Build history of the part. All positions in model axes, mm. Face numbers are marked on the shaded views. A direction names the side the tool comes from. Round coordinates to 2 decimals unless told otherwise and drop trailing zeros. Loops run counter-clockwise (first coordinate to the right, second up) from the corner with the lowest first, then second, coordinate; pieces in that order, holes last. Notation, with made-up numbers: M 21,-9 L 28,-9 A36 cw 28,27 Z; hole C 8.5,-35 d3. An arc over 180 degrees is marked long. One line per item, written item: value.
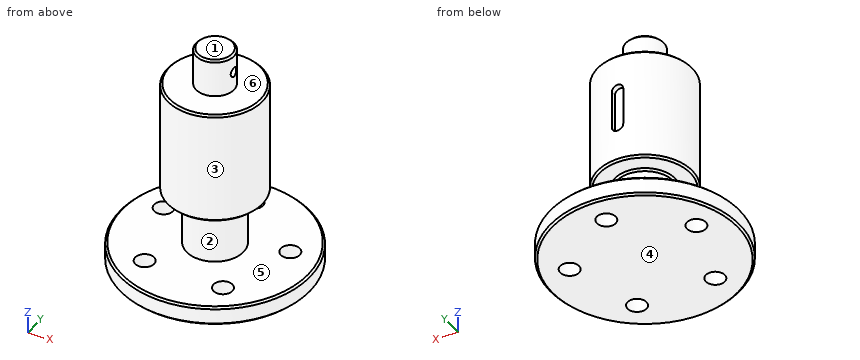
```python
from build123d import *

# Parameters (mm, degrees)
SKETCH_1_R              = 50
EXTRUDE_1_DEPTH         = 10
SKETCH_2_R              = 15
EXTRUDE_2_DEPTH         = 28
SKETCH_3_R              = 16
EXTRUDE_3_DEPTH         = 2
SKETCH_4_R              = 25
EXTRUDE_4_DEPTH         = 60
SKETCH_5_R              = 10
EXTRUDE_5_DEPTH         = 20
CHAMFER_1_SIZE          = 1
HOLE_WIZARD_10_0_10_1_D = 10
CUT_EXTRUDE_1_DEPTH     = 3
HOLE_WIZARD_5_0_5_1_D   = 5


# Read off the part's stored shape, not the designer's step: 구배27
with BuildPart() as part:
    # 스케치1 → 보스-돌출1 (new body)
    with BuildSketch(Plane.XY):
        Circle(SKETCH_1_R)
    extrude(amount=EXTRUDE_1_DEPTH)

    # 스케치2 → 보스-돌출2 (add)
    with BuildSketch(Plane.XY.offset(10)):
        Circle(SKETCH_2_R)
    extrude(amount=EXTRUDE_2_DEPTH)

    # 스케치3 → 보스-돌출3 (add)
    with BuildSketch(Plane.XY.offset(38)):
        Circle(SKETCH_3_R)
    extrude(amount=EXTRUDE_3_DEPTH)

    # 스케치4 → 보스-돌출4 (add)
    with BuildSketch(Plane.XY.offset(40)):
        Circle(SKETCH_4_R)
    extrude(amount=EXTRUDE_4_DEPTH)

    # 스케치5 → 보스-돌출5 (add)
    with BuildSketch(Plane.XY.offset(100)):
        Circle(SKETCH_5_R)
    extrude(amount=EXTRUDE_5_DEPTH)

    # 모따기1
    chamfer_1_edges = [part.edges().sort_by_distance(p)[0] for p in [
        (-25, 0, 40),
        (-25, 0, 100),
        (-50, 0, 0),
        (-10, 0, 120),
        (-50, 0, 10),
    ]]
    chamfer(chamfer_1_edges, length=CHAMFER_1_SIZE)

    # 구배27 outline → 구배27 (revolve, cut)
    with BuildSketch(Plane.XZ):
        Polygon((16, 40), (15, 39), (15, 38), (16, 38), align=None)
    revolve(axis=Axis((0, 0, 0), (0, 0, 1)), mode=Mode.SUBTRACT)

    # Ø10.0 (10) 지름 구멍1 (through all)
    with Locations(Plane(origin=(0, 0, 0), x_dir=(-1, 0, 0), z_dir=(0, 0, -1))):
        with Locations((0, 35), (-33.28697807, 10.815594803), (-20.57248383, -28.315594803), (20.57248383, -28.315594803), (33.28697807, 10.815594803)):
            Hole(HOLE_WIZARD_10_0_10_1_D / 2)

    # 스케치17 → 컷-돌출1 (cut)
    with BuildSketch(Plane(origin=(0, 25, 0), x_dir=(1, 0, 0), z_dir=(0, 1, 0))):
        with BuildLine():
            Line((-3, -60), (-3, -80))
            ThreePointArc((-3, -80), (0, -83), (3, -80))
            Line((3, -80), (3, -60))
            ThreePointArc((3, -60), (0, -57), (-3, -60))
        make_face()
    extrude(amount=-CUT_EXTRUDE_1_DEPTH, mode=Mode.SUBTRACT)

    # Ø5.0 (5) 지름 구멍1 (through all)
    with Locations(Plane(origin=(-10, 0, 0), x_dir=(0, 0, -1), z_dir=(-1, 0, 0))):
        with Locations((-110, 0)):
            Hole(HOLE_WIZARD_5_0_5_1_D / 2)


solid = part.part
```
Item 1: Which spindle directions (+Z, -Z, +X, -X, +Y, -Y) get a long thin tool onto all of the face, cutting with end or side? Do the marked faces 1, 2 and 3. Say none if no direction does.
Check values:
face 1: +Z, +X, -X, +Y, -Y
face 2: none
face 3: +Z
Item 2: Drop flat-ended pins along their axis: P1, Ø2, axis at x = 21, y = 23, coming from the +Z side; P2, Ø1, axis at y = 8.5, z = 37, coming from the +X side; P3, Ø4, axis at x = -2, y = -36.5, coming from the -Z side; P4, Ø2, axis at y = -10, z = 64.5, coming from the -X side. Give the stop position or say it passes through.
Check values:
P1: stops at z = 10
P2: stops at x = 12.69
P3: stops at z = 0
P4: stops at x = -23.32
Item 3: Wall check: line 1 along Y through (x, z) = (-0.5, 110); line 2 along Y through (x, z) = (0, 7.25); line 3 along Z through (x, y) = (-16, -23). Give the ranges that are in metal, low to high.
Check values:
line 1: y = -9.99 to -2.5, 2.5 to 9.99
line 2: y = -50 to 30, 40 to 50
line 3: z = 0 to 10
Item 4: Pull direction Z, two halves, no side cores. Call the marked faces 4, 5 and 6: pulls with the +Z half, pulls with the -Z half, needs draft (parallel to the pull), parting line crosses it, or undercut.
Check values:
face 4: pulls with the -Z half
face 5: undercut
face 6: pulls with the +Z half
Item 5: Slice it at B-B, the plane x = 0. Give the number of separate pieces and of enclosed holes in the cut face, and give its area (3 significant figures).
Check values:
separate pieces: 2
enclosed holes: 1
area: 5,100 mm2
Item 6: Slice it at C-C, the plane z = 46. Give the cut face in (x, y), and give its area (3 significant figures).
Check values:
outline: C 0,0 d50
area: 1,960 mm2
